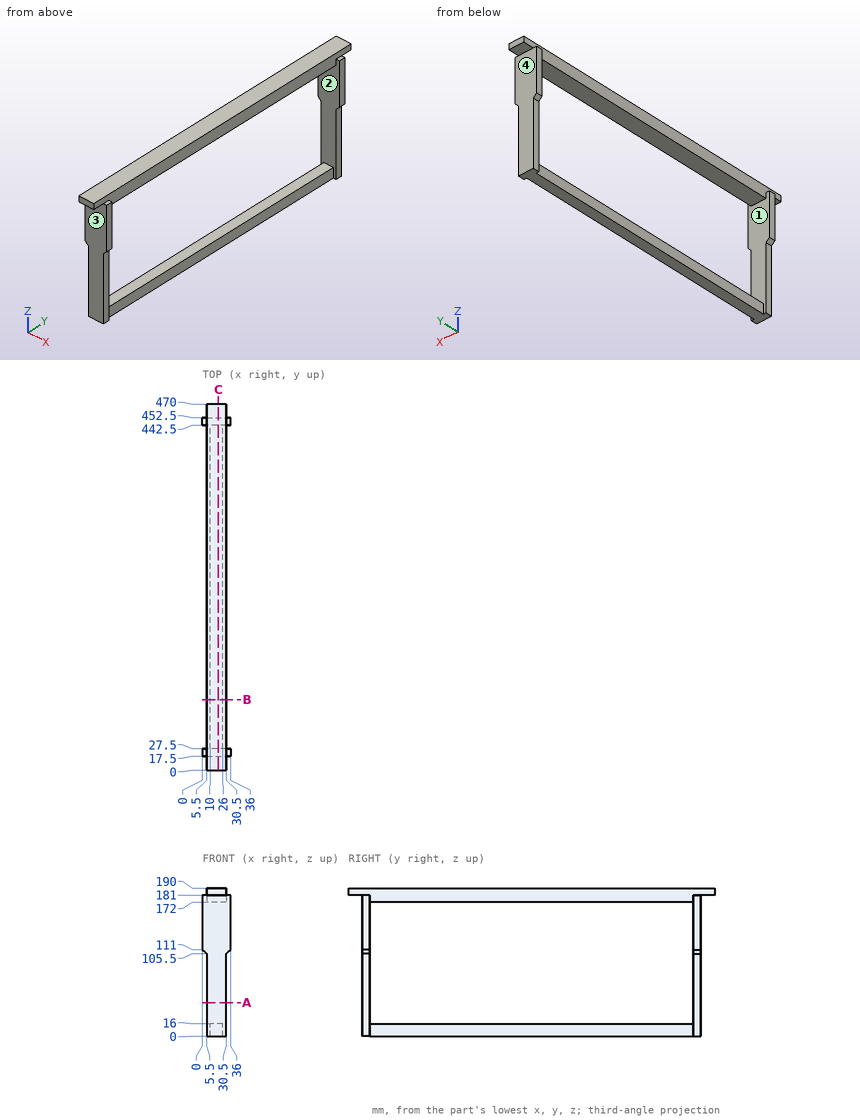
Study the drawing (mm; zero at the part's minimum x, y, z) and answer. Round coordinates to 2 decimals unless told otherwise and drop trailing zeros. Write each loop counter-clockwise with the first axis right and the second up, starting at its lowest first coordinate (ties: lowest second). Pieces come first, ordered by that corner, then holes. Notation, with made-up numbers: (-11.5, 17) -> (34.5, 17) arc R9 cw to (34.5, 21) -> close; hole circle Ø3 at (-27, 8.5). An arc over 180 degrees is marked (long way). Write each question's results on one line, items separated by ' | '.
Item 1: A cutting plane is placed at B-B, the plane y = 90.5. Determine the outline of the cut face in (x, z).
Result set:
outline: (5.5, 172) -> (30.5, 172) -> (30.5, 190) -> (5.5, 190) -> close; (10, 0) -> (26, 0) -> (26, 16) -> (10, 16) -> close
Item 2: Flat-ended cylindrical pins translate along their axes: P1, Ø8, axis at y = 165.5, z = 12, coming from the -X side; P2, Ø4, axis at x = 19, z = 156, coming from the +Y side; P3, Ø5.5, axis at y = 285, z = 177.5, coming from the +X side. Find the tip coordinate at first contact, or state that the pin passes through.
Result set:
P1: x = 10 | P2: y = 452.5 | P3: x = 30.5
Item 3: A cutting plane is placed at A-A, the plane z = 43. Determine the outline of the cut face in (x, y).
Result set:
outline: (5.5, 17.5) -> (30.5, 17.5) -> (30.5, 27.5) -> (5.5, 27.5) -> close; (5.5, 442.5) -> (30.5, 442.5) -> (30.5, 452.5) -> (5.5, 452.5) -> close
Item 4: The mould has two halves that part along Y. Classify the marked faces 1, 2, 3 and 4: +Y half, -Y half, draft (parallel to the pull), parting line (faces both ways), or undercut.
Result set:
face 1: undercut | face 2: undercut | face 3: -Y half | face 4: +Y half
Item 5: Find the intervals of material crossed by line 1 along Z through (x, y) = (23, 301); line 2 along Y through (x, z) = (29.5, 127.5); line 3 along Z through (x, y) = (6.5, 298.5), in increasing order. Write a range as [from, to].
Result set:
line 1: [0, 16], [172, 190] | line 2: [17.5, 27.5], [442.5, 452.5] | line 3: [172, 190]
Item 6: A cutting plane is placed at C-C, the plane x = 20.5. Determine the outline of the cut face in (y, z).
Result set:
outline: (0, 181) -> (17.5, 181) -> (17.5, 0) -> (452.5, 0) -> (452.5, 181) -> (470, 181) -> (470, 190) -> (0, 190) -> close; hole (27.5, 16) -> (442.5, 16) -> (442.5, 172) -> (27.5, 172) -> close
